```python
from build123d import *

# Parameters (mm, degrees)
SKETCH_1_W          = 55
SKETCH_1_H          = 35
EXTRUDE_1_DEPTH     = 37
SKETCH_3_W          = 26
SKETCH_3_H          = 32
CUT_EXTRUDE_1_DEPTH = 32
CUT_EXTRUDE_2_REACH = 76.96
SKETCH_4_R          = 0.75
CUT_EXTRUDE_3_REACH = 76.96
SKETCH_5_R          = 0.75
SKETCH_6_W          = 17
SKETCH_6_H          = 1.5
CUT_EXTRUDE_4_DEPTH = 27
SKETCH_7_R          = 18
CUT_EXTRUDE_5_DEPTH = 75.959989328


with BuildPart() as part:
    # 草图1 → 凸台-拉伸1 (new body)
    with BuildSketch(Plane.XY):
        with Locations((27.5, 17.5)):
            Rectangle(SKETCH_1_W, SKETCH_1_H)
    extrude(amount=EXTRUDE_1_DEPTH)

    # 草图3 → 切除-拉伸1 (cut)
    with BuildSketch(Plane.XZ):
        with Locations((13, 18.5)):
            Rectangle(SKETCH_3_W, SKETCH_3_H)
    extrude(amount=-CUT_EXTRUDE_1_DEPTH, mode=Mode.SUBTRACT)

    # 草图4 → 切除-拉伸2 (cut, up to next)
    with BuildSketch(Plane.XY.offset(37), mode=Mode.PRIVATE) as cut_extrude_2_sk1:
        with Locations((2, 2)):
            Circle(SKETCH_4_R)
    cut_extrude_2_tool1 = extrude(cut_extrude_2_sk1.sketch, amount=-CUT_EXTRUDE_2_REACH, mode=Mode.PRIVATE) & part.part
    # 草图4 → 切除-拉伸2 (cut, up to next)
    with BuildSketch(Plane.XY.offset(37), mode=Mode.PRIVATE) as cut_extrude_2_sk2:
        with Locations((22.5, 2)):
            Circle(SKETCH_4_R)
    cut_extrude_2_tool2 = extrude(cut_extrude_2_sk2.sketch, amount=-CUT_EXTRUDE_2_REACH, mode=Mode.PRIVATE) & part.part
    # 草图4 → 切除-拉伸2 (cut, up to next)
    with BuildSketch(Plane.XY.offset(37), mode=Mode.PRIVATE) as cut_extrude_2_sk3:
        with Locations((22.5, 22.7)):
            Circle(SKETCH_4_R)
    cut_extrude_2_tool3 = extrude(cut_extrude_2_sk3.sketch, amount=-CUT_EXTRUDE_2_REACH, mode=Mode.PRIVATE) & part.part
    # 草图4 → 切除-拉伸2 (cut, up to next)
    with BuildSketch(Plane.XY.offset(37), mode=Mode.PRIVATE) as cut_extrude_2_sk4:
        with Locations((2, 22.7)):
            Circle(SKETCH_4_R)
    cut_extrude_2_tool4 = extrude(cut_extrude_2_sk4.sketch, amount=-CUT_EXTRUDE_2_REACH, mode=Mode.PRIVATE) & part.part
    add(cut_extrude_2_tool1.solids().sort_by_distance((2, 2, 37))[0], mode=Mode.SUBTRACT)
    add(cut_extrude_2_tool2.solids().sort_by_distance((22.5, 2, 37))[0], mode=Mode.SUBTRACT)
    add(cut_extrude_2_tool3.solids().sort_by_distance((22.5, 22.7, 37))[0], mode=Mode.SUBTRACT)
    add(cut_extrude_2_tool4.solids().sort_by_distance((2, 22.7, 37))[0], mode=Mode.SUBTRACT)

    # 草图5 → 切除-拉伸3 (cut, up to next)
    with BuildSketch(Plane(origin=(0, 0, 0), x_dir=(-1, 0, 0), z_dir=(0, 0, -1)), mode=Mode.PRIVATE) as cut_extrude_3_sk1:
        with Locations(Location((-22.5, 2, 0), (0, 0, 180))):
            Circle(SKETCH_5_R)
    cut_extrude_3_tool1 = extrude(cut_extrude_3_sk1.sketch, amount=-CUT_EXTRUDE_3_REACH, mode=Mode.PRIVATE) & part.part
    # 草图5 → 切除-拉伸3 (cut, up to next)
    with BuildSketch(Plane(origin=(0, 0, 0), x_dir=(-1, 0, 0), z_dir=(0, 0, -1)), mode=Mode.PRIVATE) as cut_extrude_3_sk2:
        with Locations(Location((-2, 2, 0), (0, 0, 180))):
            Circle(SKETCH_5_R)
    cut_extrude_3_tool2 = extrude(cut_extrude_3_sk2.sketch, amount=-CUT_EXTRUDE_3_REACH, mode=Mode.PRIVATE) & part.part
    # 草图5 → 切除-拉伸3 (cut, up to next)
    with BuildSketch(Plane(origin=(0, 0, 0), x_dir=(-1, 0, 0), z_dir=(0, 0, -1)), mode=Mode.PRIVATE) as cut_extrude_3_sk3:
        with Locations((-2, 26.45)):
            Circle(SKETCH_5_R)
    cut_extrude_3_tool3 = extrude(cut_extrude_3_sk3.sketch, amount=-CUT_EXTRUDE_3_REACH, mode=Mode.PRIVATE) & part.part
    # 草图5 → 切除-拉伸3 (cut, up to next)
    with BuildSketch(Plane(origin=(0, 0, 0), x_dir=(-1, 0, 0), z_dir=(0, 0, -1)), mode=Mode.PRIVATE) as cut_extrude_3_sk4:
        with Locations((-22.5, 26.45)):
            Circle(SKETCH_5_R)
    cut_extrude_3_tool4 = extrude(cut_extrude_3_sk4.sketch, amount=-CUT_EXTRUDE_3_REACH, mode=Mode.PRIVATE) & part.part
    add(cut_extrude_3_tool1.solids().sort_by_distance((22.5, 2, 0))[0], mode=Mode.SUBTRACT)
    add(cut_extrude_3_tool2.solids().sort_by_distance((2, 2, 0))[0], mode=Mode.SUBTRACT)
    add(cut_extrude_3_tool3.solids().sort_by_distance((2, 26.45, 0))[0], mode=Mode.SUBTRACT)
    add(cut_extrude_3_tool4.solids().sort_by_distance((22.5, 26.45, 0))[0], mode=Mode.SUBTRACT)

    # 草图6 → 切除-拉伸4 (cut)
    with BuildSketch(Plane.XZ):
        with Locations((12.25, 35.25)):
            Rectangle(SKETCH_6_W, SKETCH_6_H)
    extrude(amount=-CUT_EXTRUDE_4_DEPTH, mode=Mode.SUBTRACT)

    # 草图7 → 切除-拉伸5 (cut, through all)
    with BuildSketch(Plane.XY.offset(37)):
        Circle(SKETCH_7_R)
    extrude(amount=-CUT_EXTRUDE_5_DEPTH, mode=Mode.SUBTRACT)


solid = part.part
```
Geometry check sheet. Reference: the model listing, model coordinates, mm. A direction names the side the tool comes from. Round coordinates to 2 decimals unless told otherwise and drop trailing zeros. Loops run counter-clockwise (first coordinate to the right, second up) from the corner with the lowest first, then second, coordinate; pieces in that order, holes last. Notation, with made-up numbers: (65, 33) - (104, 33) arc R18 cw to (104, 42) - close; hole circle Ø4 at (28, 11). An arc over 180 degrees is marked (long way). Write item = value, one per line. Start each with the question number.
1. Section check A-A on x = 22.5. Enter the section's corners in (y, z), then the cut area to 3 significant figures.
2. Set-up check for faces 1 (the face through (20.75, 13, 35)), 2 (the face through (26, 16, 18)), 3 (the face through (2.69, 22.41, 35.77)): record each of +Z, -Z, +X, -X, +Y, -Y from which the full face is reachable in a straight line by a thin tool's end or side.
3. Mould release check, pull along Y, two halves, no side actions. Record for faces 4 (the face through (21.75, 1.97, 1.23)), 5 (the face through (14, 19, 36)), 6 (the face through (12.867, 12.587, 1.267)): released by +Y, released by -Y, zero draft, split by the parting line, or undercut.
4. Section check B-B on y = 22.7. Enter the section's corners in (x, z).
5. Thickness scan on line 1 (Y direction, x = 22.5, z = 0.85); line 2 (Y direction, x = 22.5, z = 35.45); line 3 (Y direction, x = 20.5, z = 32.5). Record the ranges inside material, lowest first.
6. Depth check by flat-ended pin: pin 1 (0.8 mm diameter, centred on y = 16, z = 35, fed in from -X); pin 2 (18.5 mm diameter, centred on x = 13.5, y = 15.5, fed in from -Z); pin 3 (13 mm diameter, centred on x = 10.5, z = 17, fed in from -Y); pin 4 (12 mm diameter, centred on y = 6.5, z = 11.5, fed in from -X). Enter the tip coordinate at first touch or a pass-through.
7. Section check D-D on y = 19. Enter the section's corners in (x, z), then the cut area to 3 significant figures.
8. Section check C-C on x = 2. Enter the section's corners in (y, z), then the cut area to 3 significant figures.
Working result:
q1.outline = (0, 0) - (1.25, 0) - (1.25, 2.5) - (0, 2.5) - close; (0, 34.5) - (1.25, 34.5) - (1.25, 37) - (0, 37) - close; (2.75, 0) - (25.7, 0) - (25.7, 2.5) - (2.75, 2.5) - close; (2.75, 34.5) - (21.95, 34.5) - (21.95, 37) - (2.75, 37) - close; (23.45, 34.5) - (32, 34.5) - (32, 2.5) - (27.2, 2.5) - (27.2, 0) - (35, 0) - (35, 37) - (23.45, 37) - close
q1.area = 256 mm^2
q2.face_1 = -Y
q2.face_2 = -X, -Y
q2.face_3 = +Z
q3.face_4 = undercut
q3.face_5 = zero draft
q3.face_6 = released by -Y
q4.outline = (0, 0) - (55, 0) - (55, 37) - (23.25, 37) - (23.25, 34.5) - (26, 34.5) - (26, 2.5) - (0, 2.5) - close; (0, 34.5) - (1.25, 34.5) - (1.25, 37) - (0, 37) - close; (2.75, 34.5) - (3.75, 34.5) - (3.75, 36) - (20.75, 36) - (20.75, 34.5) - (21.75, 34.5) - (21.75, 37) - (2.75, 37) - close
q5.line_1 = 0 to 1.25, 2.75 to 25.7, 27.2 to 35
q5.line_2 = 0 to 1.25, 2.75 to 21.95, 23.45 to 35
q5.line_3 = 32 to 35
q6.pin_1 = 20.75
q6.pin_2 = 0
q6.pin_3 = 32
q6.pin_4 = 26
q7.outline = (0, 0) - (55, 0) - (55, 37) - (0, 37) - (0, 34.5) - (3.75, 34.5) - (3.75, 36) - (20.75, 36) - (20.75, 34.5) - (26, 34.5) - (26, 2.5) - (0, 2.5) - close
q7.area = 1,180 mm^2
q8.outline = (17.89, 0) - (25.7, 0) - (25.7, 2.5) - (17.89, 2.5) - close; (17.89, 34.5) - (21.95, 34.5) - (21.95, 37) - (17.89, 37) - close; (23.45, 34.5) - (32, 34.5) - (32, 2.5) - (27.2, 2.5) - (27.2, 0) - (35, 0) - (35, 37) - (23.45, 37) - close
q8.area = 174 mm^2
